from build123d import *

# Parameters (mm, degrees)
SKETCH1_R           = 2.5
BOSS_EXTRUDE1_DEPTH = 3
SKETCH2_R           = 6
BOSS_EXTRUDE2_DEPTH = 2
FILLET1_R           = 1


with BuildPart() as part:
    # Sketch1 → Boss-Extrude1 (new body)
    with BuildSketch(Plane(origin=(0, 0, 0), x_dir=(1, 0, 0), z_dir=(0, 1, 0))):
        with Locations(Location((0, 0, 0), (0, 0, 270))):
            Circle(SKETCH1_R)
    extrude(amount=BOSS_EXTRUDE1_DEPTH)

    # Sketch2 → Boss-Extrude2 (add)
    with BuildSketch(Plane(origin=(0, 3, 0), x_dir=(1, 0, 0), z_dir=(0, 1, 0))):
        with Locations(Location((0, 0, 0), (0, 0, 270))):
            Circle(SKETCH2_R)
    extrude(amount=BOSS_EXTRUDE2_DEPTH)

    # Fillet1
    fillet1_edges = [part.edges().sort_by_distance(p)[0] for p in [
        (0, 3, -6),
        (0, 5, -6),
    ]]
    fillet(fillet1_edges, radius=FILLET1_R - 0.0001)  # a hair under: the kernel refuses the full size

    # Mirror1: part across plane


with BuildPart() as part_1:
    add(part.part)
    add(part.part.mirror(Plane.ZX))


solid = part_1.part
Verification items for the finished model (mm, model axes). Give positions to 0.01 mm unless a question says otherwise; leave off trailing zeros. Loops run counter-clockwise (first coordinate to the right, second up) from the corner with the lowest first, then second, coordinate; pieces in that order, holes last.
1. Go/stop test with flat-tipped pins: P1, Ø1, axis at y = 1.5, z = -0.5, coming from the +X side; P2, Ø6, axis at x = -4, y = -2.5, coming from the -Z side. Record where each tip stops, or that it passes through.
Derived:
P1: stops at x = 2.5
P2: stops at z = -5.84
2. Material ranges on probe 1 along Y at (x, z) = (-1.25, 4); probe 2 along Y at (x, z) = (5, -2.5); probe 3 along X at (y, z) = (-3.25, 4.5), recorded low to high.
Derived:
probe 1: y = -5 to -3, 3 to 5
probe 2: y = -4.81 to -3.19, 3.19 to 4.81
probe 3: x = -3.44 to 3.44
3. Cross-section at C-C on y = 2.25. Record the cut outline in (x, z).
Derived:
outline: circle Ø5 at (0, 0)
4. Cross-section at D-D on y = 3.5. Record the cut outline in (x, z), and give its area (3 significant figures).
Derived:
outline: circle Ø11.73 at (0, 0)
area: 108 mm2
5. Release check for a two-part mould opening along Y. For faces 1 (the flat face through (0, -5, 0)), 2 (the cylindrical face through (-2.44, 0.04, -0.54)), 3 (the flat face through (-2, -3, 2)), 4 (the flat face through (0, 5, 0)) record: +Y half, -Y half, draft (parallel to the pull), parting line (faces both ways), or undercut.
Derived:
face 1: -Y half
face 2: undercut
face 3: undercut
face 4: +Y half
